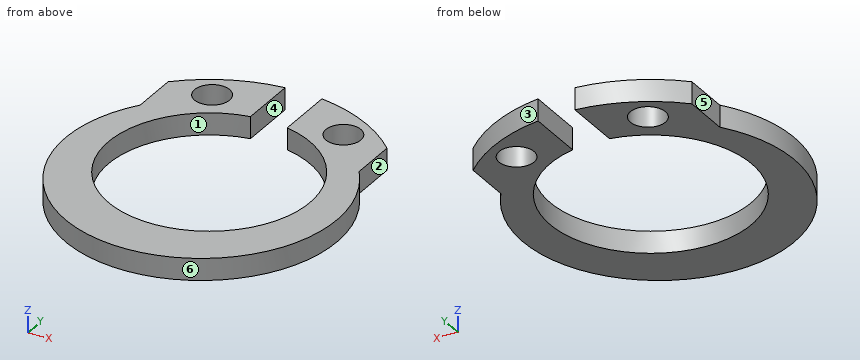
from build123d import *

# Parameters (mm, degrees)
F0_R     = 0.4
F1_DEPTH = 0.5
F2_SCALE = 3


with BuildPart() as f1:
    # F0 (on Top) → F1 (new body)
    with BuildSketch(Plane.XY):
        with BuildLine():
            Line((2.5, 1.533030278), (2.5, 2.5903667694))
            ThreePointArc((2.5, 2.5903667694), (1.5408376054, 3.2535856334), (0.42, 3.5754160597))
            Line((0.42, 3.5754160597), (0.42, 2.261327044))
            ThreePointArc((0.42, 2.261327044), (0, -2.3), (-0.42, 2.261327044))
            Line((-0.42, 2.261327044), (-0.42, 3.5754160597))
            ThreePointArc((-0.42, 3.5754160597), (-1.5408376054, 3.2535856334), (-2.5, 2.5903667694))
            Line((-2.5, 2.5903667694), (-2.5, 1.533030278))
            ThreePointArc((-2.5, 1.533030278), (0, -3.4), (2.5, 1.533030278))
        make_face()
        with Locations((-1.5, 2.5980762114)):
            Circle(F0_R, mode=Mode.SUBTRACT)
        with Locations((1.5, 2.5980762114)):
            Circle(F0_R, mode=Mode.SUBTRACT)
    extrude(amount=F1_DEPTH)


with BuildPart() as f1_1:
    # F2: moved
    add(f1.part.scale(F2_SCALE))


solid = f1_1.part
Design review of the part built by this model. Coordinates are the model's own, in mm. Face numbers are marked on the shaded views. A direction names the side the tool comes from. Coordinates: 2 decimals unless noted, no trailing zeros. Order: outer loops, then holes, each group sorted by start corner. A loop starts at its lowest first (then second) coordinate and runs counter-clockwise, first axis right, second up. Notation, with made-up numbers: (18.25, -6.5) -> (29.25, -6.5) arc R33 cw to (29.25, 30.5) -> close; hole circle Ø3 at (-10, 11.25). An arc over 180 degrees is marked (long way). One line per item, written item: value.
1) We need section B-B, the plane x = 2.25. Give the boundary of the cut face in (y, z).
Output values:
outline: (-9.92, 0) -> (-6.52, 0) -> (-6.52, 1.5) -> (-9.92, 1.5) -> close; (6.52, 0) -> (10.56, 0) -> (10.56, 1.5) -> (6.52, 1.5) -> close
2) Machinability: for the marked faces 4, 5 and 6, which of the approach directions +Z, -Z, +X, -X, +Y, -Y give a long, thin tool a straight path to every point of the face, cutting with its end or side? Answer none if there is none.
Output values:
face 4: +Z, -Z, +Y
face 5: +Z, -Z, -X, +Y
face 6: +Z, -Z
3) We need section C-C, the plane x = 5. Give the boundary of the cut face in (y, z) (3 decimals), then the cut area to 3 significant figures.
Output values:
outline: (-8.742, 0) -> (-4.755, 0) -> (-4.755, 1.5) -> (-8.742, 1.5) -> close; (4.755, 0) -> (6.703, 0) -> (6.703, 1.5) -> (4.755, 1.5) -> close; (8.885, 0) -> (9.573, 0) -> (9.573, 1.5) -> (8.885, 1.5) -> close
area: 9.93 mm2
4) To check wall thickness, follow probe 1 along X at (y, z) = (8, 0.8); probe 2 along X at (y, z) = (-3.5, 0.45); probe 3 along Y at (x, z) = (4.5, 1.25). State the ranges of each line that lie inside material, in increasing order. Write a range as [from, to].
Output values:
probe 1: x = [-7.26, -5.68], [-3.32, -1.26], [1.26, 3.32], [5.68, 7.26]
probe 2: x = [-8.93, -5.95], [5.95, 8.93]
probe 3: y = [-9.04, -5.23], [5.23, 6.59], [8.99, 9.82]
5) Draft analysis for pull direction Y (two halves, no side actions). For the marked faces 1, 2 and 3, state which applies: +Y half, -Y half, draft (parallel to the pull), parting line (faces both ways), or undercut.
Output values:
face 1: undercut
face 2: draft
face 3: +Y half
6) We need section D-D, the plane y = 7.5. Give the boundary of the cut face in (x, z), then the cut area to 3 significant figures.
Output values:
outline: (-7.5, 0) -> (-5.66, 0) -> (-5.66, 1.5) -> (-7.5, 1.5) -> close; (-3.34, 0) -> (-1.26, 0) -> (-1.26, 1.5) -> (-3.34, 1.5) -> close; (1.26, 0) -> (3.34, 0) -> (3.34, 1.5) -> (1.26, 1.5) -> close; (5.66, 0) -> (7.5, 0) -> (7.5, 1.5) -> (5.66, 1.5) -> close
area: 11.7 mm2
7) We need section A-A, the plane y = -0.75. Give the boundary of the cut face in (x, z).
Output values:
outline: (-9.3, 0) -> (-6.86, 0) -> (-6.86, 1.5) -> (-9.3, 1.5) -> close; (6.86, 0) -> (9.3, 0) -> (9.3, 1.5) -> (6.86, 1.5) -> close
